Geometry check sheet. Reference: the model listing, model coordinates, mm. Face numbers are marked on the shaded views. A direction names the side the tool comes from. Give positions to 0.01 mm unless a question says otherwise; leave off trailing zeros. Write each loop counter-clockwise with the first axis right and the second up, starting at its lowest first coordinate (ties: lowest second). Pieces come first, ordered by that corner, then holes. Notation, with made-up numbers: M 81,62 L 139,62 A33 cw 139,93 Z; hole C -36,82 d6. An arc over 180 degrees is marked long. One line per item, written item: value. Start each with the question number.
1. Cross-section at B-B on y = 126.5. Record the cut outline in (x, z), then the cut area to 3 significant figures.
2. Release check for a two-part mould opening along Y. For the marked faces 3, 4 and 5 record: pulls with the +Y half, pulls with the -Y half, needs draft (parallel to the pull), parting line crosses it, or undercut.
3. Tool access check on the marked faces 1 and 2. Record the directions out of +Z, -Z, +X, -X, +Y, -Y that give a thin tool (end or side, any length) a straight path to the whole face; none if there is none.
4. Gauge pin test, flat ends, axial feed: pin 1 (5 mm diameter, centred on y = 267.5, z = 71.5, fed in from +X); pin 2 (8 mm diameter, centred on x = -110.5, y = -40.5, fed in from +Z). Record the tip position at first contact, or that the pin passes through.
5. Cross-section at C-C on x = 130.5. Record the cut outline in (y, z).
6. Cross-section at D-D on x = -43.5. Record the cut outline in (y, z).
7. Cross-section at A-A on z = 44. Record the cut outline in (x, y).
8. Scan lines: line 1 (Y direction, x = 256, z = 82); line 2 (Y direction, x = -40, z = 89.5); line 3 (X direction, y = -47, z = 58.5). Record each from-to range of solid material in increasing order.
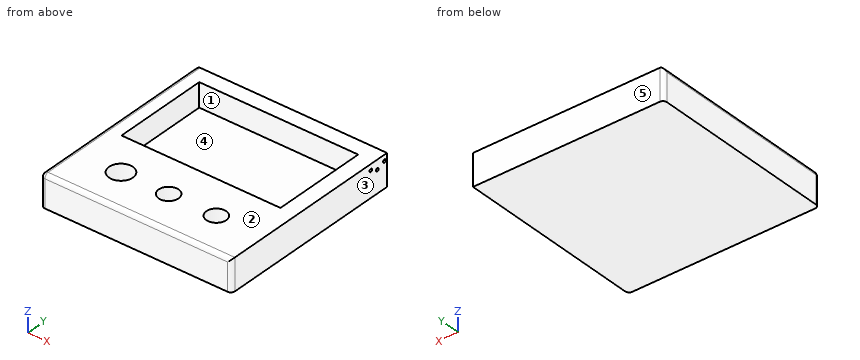
from build123d import *

# Parameters (mm, degrees)
F0_W     = 609.6
F0_H     = 609.6
F1_DEPTH = 101.6
F2_W     = 508
F2_H     = 304.8
F2_R     = 38.1
F2_R_2   = 31.75
F3_DEPTH = 76.2
F4_R     = 12.7
F5_R     = 5.08
F6_DEPTH = 38.1


with BuildPart() as f1:
    # F0 (on Top) → F1 (new body)
    with BuildSketch(Plane.XY):
        with Locations((-38.065076, 1.158021)):
            Rectangle(F0_W, F0_H)
    extrude(amount=F1_DEPTH)

    # F2 (on face) → F3 (cut)
    with BuildSketch(Plane.XY.offset(101.6)):
        with Locations((-38.065076, 102.758021)):
            Rectangle(F2_W, F2_H)
        with Locations((-190.465076, -176.641979)):
            Circle(F2_R)
        with Locations((-38.065076, -176.641979)):
            Circle(F2_R_2)
        with Locations((114.334924, -176.641979)):
            Circle(F2_R_2)
    extrude(amount=-F3_DEPTH, mode=Mode.SUBTRACT)

    # F4
    f4_edges = [f1.edges().sort_by_distance(p)[0] for p in [
        (-38.065076, -303.641979, 101.6),
        (266.734924, -303.641979, 50.8),
        (-342.865076, 1.158021, 101.6),
        (-342.865076, -303.641979, 50.8),
        (-342.865076, 305.958021, 50.8),
    ]]
    fillet(f4_edges, radius=F4_R)

    # F5 (on face) → F6 (cut)
    with BuildSketch(Plane.YZ.offset(266.734924)):
        with Locations((242.362949, 82.55)):
            Circle(F5_R)
        with Locations((267.858021, 71.12)):
            Circle(F5_R)
        with Locations((295.798021, 82.55)):
            Circle(F5_R)
    extrude(amount=-F6_DEPTH, mode=Mode.SUBTRACT)


solid = f1.part
Report:
1. outline: M -342.87,0 L 266.73,0 L 266.73,101.6 L 215.93,101.6 L 215.93,25.4 L -292.07,25.4 L -292.07,101.6 L -330.17,101.6 A12.7 ccw -342.87,88.9 Z
1. area: 23,200 mm^2
2. face 3: needs draft
2. face 4: undercut
2. face 5: pulls with the +Y half
3. face 1: +Z
3. face 2: +Z, +X, -X, +Y, -Y
4. pin 1: stops at x = 228.63
4. pin 2: stops at z = 25.4
5. outline: M -303.64,0 L 305.96,0 L 305.96,101.6 L 255.16,101.6 L 255.16,25.4 L -49.64,25.4 L -49.64,101.6 L -149.32,101.6 L -149.32,25.4 L -203.97,25.4 L -203.97,101.6 L -290.94,101.6 A12.7 ccw -303.64,88.9 Z
6. outline: M -303.64,0 L 305.96,0 L 305.96,101.6 L 255.16,101.6 L 255.16,25.4 L -49.64,25.4 L -49.64,101.6 L -145.36,101.6 L -145.36,25.4 L -207.92,25.4 L -207.92,101.6 L -290.94,101.6 A12.7 ccw -303.64,88.9 Z
7. outline: M -342.87,-290.94 A12.7 ccw -330.17,-303.64 L 254.03,-303.64 A12.7 ccw 266.73,-290.94 L 266.73,305.96 L -330.17,305.96 A12.7 ccw -342.87,293.26 Z; hole M -292.07,-49.64 L 215.93,-49.64 L 215.93,255.16 L -292.07,255.16 Z; hole C -190.47,-176.64 d76.2; hole C -38.07,-176.64 d63.5; hole C 114.33,-176.64 d63.5
8. line 1: y = -303.49 to 237.31, 247.41 to 290.75, 300.85 to 305.96
8. line 2: y = -303.63 to -208.33, -144.95 to -49.64, 255.16 to 305.96
8. line 3: x = -342.87 to -292.07, 215.93 to 266.73
